Job drawing, mm, ordinate dimensions from the low corner. One solid piece. A direction names the side the tool comes from. Coordinates: 2 decimals unless noted, no trailing zeros. Order: outer loops, then holes, each group sorted by start corner. A loop starts at its lowest first (then second) coordinate and runs counter-clockwise, first axis right, second up. Notation, with made-up numbers: M -28,-2 L -5,-2 A31 cw -5,31 Z; hole C -38.5,12 d5. An arc over 180 degrees is marked long. Write item = value, one per line.
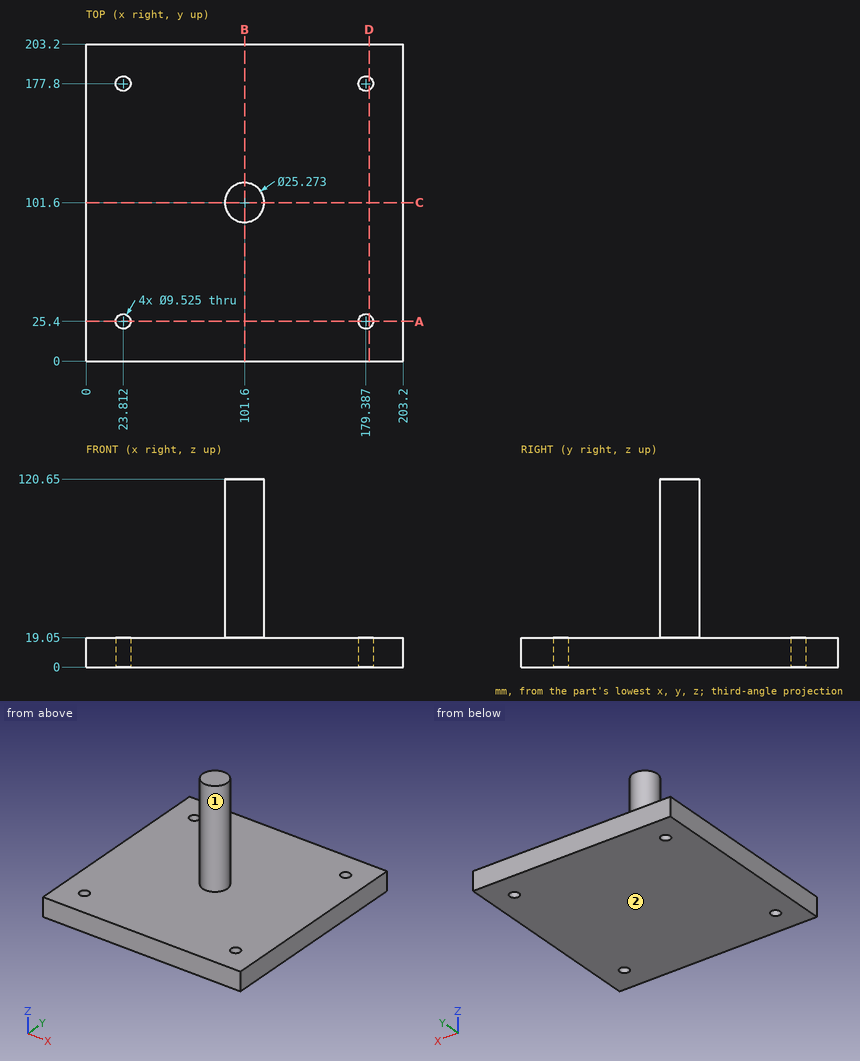
(1) Wall check: line 1 (X direction, y = 25, z = 8); line 2 (Z direction, x = 78.5, y = 48.5); line 3 (X direction, y = 177, z = 4). Give the ranges that are in metal, low to high. Write a range as from..to.
Evaluation:
line_1 = 0..19.07, 28.56..174.64, 184.13..203.2
line_2 = 0..19.05
line_3 = 0..19.12, 28.51..174.69, 184.08..203.2
(2) Tool access for the marked faces 1 and 2: list every direction of +Z, -Z, +X, -X, +Y, -Y with a clear straight run to the whole face (end or side of a thin tool).
Evaluation:
face_1 = +Z
face_2 = -Z, +X, -X, +Y, -Y
(3) Slice it at B-B, the plane x = 101.6. Write the cut outline in (y, z).
Evaluation:
outline = M 0,0 L 203.2,0 L 203.2,19.05 L 114.24,19.05 L 114.24,120.65 L 88.96,120.65 L 88.96,19.05 L 0,19.05 Z
(4) Pin check, flat tips, straight feed: pin 1 Ø2 at (y, z) = (86, 52) entering from +X; pin 2 Ø12 at (x, y) = (118, 178.5) entering from -Z; pin 3 Ø6 at (y, z) = (110.5, 74.5) entering from -X (1 decimal); pin 4 Ø11 at (x, y) = (23.81, 25.4) entering from +Z. Stop position of each tip, or through.
Evaluation:
pin_1 = through
pin_2 = 0
pin_3 = 90.4
pin_4 = 19.05
(5) Slice it at A-A, the plane y = 25.4. State how many separate pieces and enclosed holes the cut face has, then the cut area to 3 significant figures.
Evaluation:
separate_pieces = 3
enclosed_holes = 0
area = 3,510 mm²
(6) Slice it at D-D, the plane x = 181.5. Write the cut outline in (y, z), then the cut area to 3 significant figures.
Evaluation:
outline = M 0,0 L 21.13,0 L 21.13,19.05 L 0,19.05 Z; M 29.67,0 L 173.53,0 L 173.53,19.05 L 29.67,19.05 Z; M 182.07,0 L 203.2,0 L 203.2,19.05 L 182.07,19.05 Z
area = 3,550 mm²
